Verification items for the finished model (mm, model axes). Face numbers are marked on the shaded views. A direction names the side the tool comes from. Round coordinates to 2 decimals unless told otherwise and drop trailing zeros. Loops run counter-clockwise (first coordinate to the right, second up) from the corner with the lowest first, then second, coordinate; pieces in that order, holes last. Notation, with made-up numbers: M -39.5,-10 L 15.5,-10 A12 cw 15.5,-6 Z; hole C 89,-18.75 d4. An arc over 180 degrees is marked long. One line per item, written item: value.
from build123d import *

# Parameters (mm, degrees)
SKETCH_1_W          = 39
SKETCH_1_H          = 16
EXTRUDE_1_DEPTH     = 1.5
SKETCH_2_R          = 1.75
CUT_EXTRUDE_1_DEPTH = 1.5
SKETCH_3_W          = 12.5
SKETCH_3_H          = 6
EXTRUDE_2_DEPTH     = 6
SKETCH_4_W          = 10
SKETCH_4_H          = 15
EXTRUDE_3_DEPTH     = 6


with BuildPart() as part:
    # 草图1 → 凸台-拉伸1 (new body)
    with BuildSketch(Plane(origin=(0, 0, 0), x_dir=(1, 0, 0), z_dir=(0, 1, 0))):
        Rectangle(SKETCH_1_W, SKETCH_1_H)
    extrude(amount=EXTRUDE_1_DEPTH)

    # 草图2 → 切除-拉伸1 (cut)
    with BuildSketch(Plane(origin=(0, 1.5, 0), x_dir=(1, 0, 0), z_dir=(0, 1, 0))):
        with Locations(Location((16.25, 4.75, 0), (0, 0, 270))):
            Circle(SKETCH_2_R)
        with Locations(Location((-2.75, 4.75, 0), (0, 0, 270))):
            Circle(SKETCH_2_R)
    extrude(amount=-CUT_EXTRUDE_1_DEPTH, mode=Mode.SUBTRACT)

    # 草图3 → 凸台-拉伸2 (add)
    with BuildSketch(Plane(origin=(0, 1.5, 0), x_dir=(1, 0, 0), z_dir=(0, 1, 0))):
        with Locations((6.75, 5)):
            Rectangle(SKETCH_3_W, SKETCH_3_H)
    extrude(amount=EXTRUDE_2_DEPTH)

    # 草图4 → 凸台-拉伸3 (add)
    with BuildSketch(Plane(origin=(0, 1.5, 0), x_dir=(1, 0, 0), z_dir=(0, 1, 0))):
        with Locations((-14, 0)):
            Rectangle(SKETCH_4_W, SKETCH_4_H)
    extrude(amount=EXTRUDE_3_DEPTH)


solid = part.part
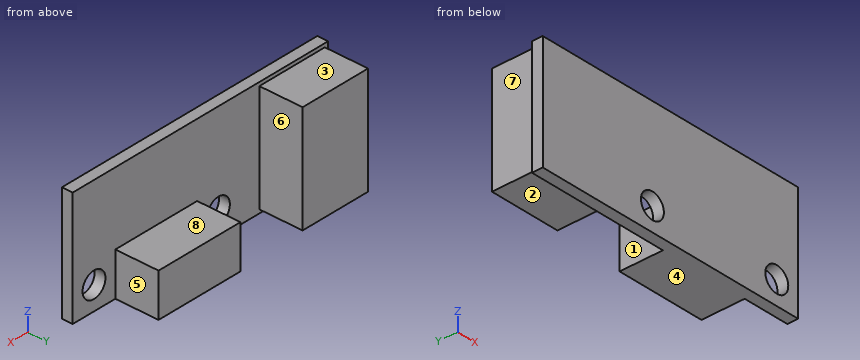
(1) Sectioned sample at D-D on z = 4. Enter the section's corners in (x, y).
Completed:
outline: M -19.5,0 L 19.5,0 L 19.5,1.5 L -9,1.5 L -9,7.5 L -19,7.5 L -19,1.5 L -19.5,1.5 Z
(2) Mould release check, pull along Z, two halves, no side actions. Record for the marked faces 1, 2 and 3: +Z half, -Z half, draft (parallel to the pull), parting line (faces both ways), or undercut.
Completed:
face 1: draft
face 2: -Z half
face 3: +Z half
(3) Depth check by flat-ended pin: pin 1 Ø1.8 at (x, y) = (-13.5, 3.5) entering from -Z; pin 2 Ø1.5 at (y, z) = (3, -1) entering from -X; pin 3 Ø3 at (y, z) = (5.5, 0) entering from +X; pin 4 Ø3 at (x, z) = (16.25, -4.75) entering from -Y. Enter the tip coordinate at first touch or a pass-through.
Completed:
pin 1: stops at z = -7.5
pin 2: stops at x = -19
pin 3: stops at x = -9
pin 4: passes through
(4) Sectioned sample at B-B on z = -4.75. Enter the section's corners in (x, y), and give its area (3 significant figures).
Completed:
outline: M -19.5,0 L -4.5,0 L -4.5,1.5 L -9,1.5 L -9,7.5 L -19,7.5 L -19,1.5 L -19.5,1.5 Z; M -1,0 L 14.5,0 L 14.5,1.5 L 13,1.5 L 13,7.5 L 0.5,7.5 L 0.5,1.5 L -1,1.5 Z; M 18,0 L 19.5,0 L 19.5,1.5 L 18,1.5 Z
area: 183 mm^2
(5) Sectioned sample at C-C on x = -12.5. Enter the section's corners in (y, z), and give its area (3 significant figures).
Completed:
outline: M 0,-8 L 1.5,-8 L 1.5,-7.5 L 7.5,-7.5 L 7.5,7.5 L 1.5,7.5 L 1.5,8 L 0,8 Z
area: 114 mm^2
(6) Sectioned sample at A-A on x = -2.75. Enter the section's corners in (y, z).
Completed:
outline: M 0,-8 L 1.5,-8 L 1.5,-6.5 L 0,-6.5 Z; M 0,-3 L 1.5,-3 L 1.5,8 L 0,8 Z
(7) Tool access check on the marked faces 4, 5, 6, 7 and 8. Record the directions out of +Z, -Z, +X, -X, +Y, -Y that give a thin tool (end or side, any length) a straight path to the whole face; none if there is none.
Completed:
face 4: -Z, +X, -X, +Y, -Y
face 5: +Z, -Z, +X, +Y
face 6: +Z, -Z, +Y
face 7: +Z, -Z, -X, +Y
face 8: +Z, +X, +Y
(8) Thickness scan on L1, parallel to X at y = 0.4, z = -4.75; L2, parallel to X at y = 3.25, z = -2.25; L3, parallel to Y at x = -4.5, z = 6.25. Record the ranges inside material, lowest first. Write a range as from..to.
Completed:
L1: x = -19.5..-4.5, -1..14.5, 18..19.5
L2: x = -19..-9, 0.5..13
L3: y = 0..1.5
